```python
from build123d import *

# Parameters (mm, degrees)
F0_R     = 3.15
F1_DEPTH = 5
F2_R     = 4.99999
F3_R     = 1


# Not quite as in the source:
# - a fillet or chamfer is up to 0.001 mm smaller than in the source, because OpenCascade refuses the exact size


with BuildPart() as f1:
    # F0 (on Top) → F1 (new body)
    with BuildSketch(Plane.XY):
        Polygon((-49.8123717308, 43.8505291194), (-54.8123717308, 43.8505291194), (-54.8123717308, 33.8505291194), (-16.8123717308, 33.8505291194), (-16.8123717308, 43.8505291194), align=None)
        with Locations((-49.8123717308, 38.8505291194)):
            Circle(F0_R, mode=Mode.SUBTRACT)
        with Locations((-21.8123717308, 38.8505291194)):
            Circle(F0_R, mode=Mode.SUBTRACT)
    extrude(amount=F1_DEPTH)

    # F2 (radius 5 in the source; OpenCascade refuses exactly that, so slightly less here)
    f2_edges = [f1.edges().sort_by_distance(p)[0] for p in [
        (-54.812372, 33.850529, 2.5),
        (-54.812372, 43.850529, 2.5),
        (-16.812372, 43.850529, 2.5),
        (-16.812372, 33.850529, 2.5),
    ]]
    fillet(f2_edges, radius=F2_R)

    # F3
    f3_edges = [f1.edges().sort_by_distance(p)[0] for p in [
        (-35.812372, 33.850529, 5),
        (-35.812372, 43.850529, 5),
    ]]
    fillet(f3_edges, radius=F3_R)


solid = f1.part
```
Can you work these out from the model? Positions are in its coordinate system, mm. Coordinates: 2 decimals unless noted, no trailing zeros. Loops run counter-clockwise (first coordinate to the right, second up) from the corner with the lowest first, then second, coordinate; pieces in that order, holes last.
1) Imagine slicing it at B-B on x = -24. List the corners of the cut face in (y, z) for me.
2) Thinking about a two-plate mould opening in X: for faces 1 (the cylindrical face through (-53, 35, 2)), 2 (the flat face through (-36, 39, 0)), 3 (the cylindrical face through (-22.222, 41.974, 2.465)), which applies, pulls with the +X half, pulls with the -X half, needs draft (parallel to the pull), parting line crosses it, or undercut?
3) I need wall thicknesses on probe 1 along X at (y, z) = (38.75, 2); probe 2 along X at (y, z) = (37.5, 0.8); probe 3 along Y at (x, z) = (-50, 1.1). Which ranges of each line are inside material? Lowest first, please.
4) Imagine slicing it at A-A on z = 3.1. State how many separate pieces and enclosed holes the cut face has, plus the area to 3 significant figures.
5) For pin 1 (5 mm diameter, centred on x = -49.81, y = 38.85, fed in from +Z), with a flat end and sliding along its axis, tell me the tip position at first contact or that it passes through.
Completed:
1. outline: (33.85, 0) - (36.58, 0) - (36.58, 5) - (34.85, 5) arc R1 ccw to (33.85, 4) - close; (41.12, 0) - (43.85, 0) - (43.85, 4) arc R1 ccw to (42.85, 5) - (41.12, 5) - close
2. face 1: pulls with the -X half
2. face 2: needs draft
2. face 3: undercut
3. probe 1: x = -54.81 to -52.96, -46.66 to -24.96, -18.66 to -16.81
3. probe 2: x = -54.63 to -52.66, -46.97 to -24.66, -18.97 to -17
3. probe 3: y = 33.85 to 35.71, 41.99 to 43.85
4. separate pieces: 1
4. enclosed holes: 2
4. area: 296 mm2
5. pin 1: passes through
